```python
from build123d import *

# Parameters (mm, degrees)
PAD_DEPTH       = 3
SKETCH001_R     = 8.6
POCKET_DEPTH    = 3.001
SKETCH002_W     = 50
SKETCH002_H     = 6
PAD001_DEPTH    = 6
SKETCH003_W     = 5
SKETCH003_H     = 4.5
POCKET001_DEPTH = 6


with BuildPart() as part:
    # Sketch → Pad (new body)
    with BuildSketch(Plane.XZ):
        with BuildLine():
            Line((-24, -25), (-24, -24))
            Line((-24, -24), (-23, -24))
            Line((-23, -24), (-23, -17))
            Line((-23, -17), (-26.5, -17))
            Line((-26.5, -17), (-26.5, -14))
            Line((-26.5, -14), (-23.5, -14))
            Line((-23.5, -14), (-23.5, 0))
            Line((-23.5, 0), (-25, 0))
            Line((-25, 0), (-25, 30))
            Line((-25, 30), (25, 30))
            Line((25, 30), (25, 0))
            Line((25, 0), (23.5, 0))
            Line((23.5, 0), (23.5, -14))
            Line((23.5, -14), (26.5, -14))
            Line((26.5, -14), (26.5, -17))
            Line((26.5, -17), (23, -17))
            Line((23, -17), (23, -24))
            Line((23, -24), (24, -24))
            Line((24, -24), (24, -25))
            ThreePointArc((19, -21), (20.983324, -23.645845), (24, -25))
            Line((19, -3), (19, -21))
            Line((14, -3), (19, -3))
            Line((14, -18), (14, -3))
            Line((-14, -18), (14, -18))
            Line((-14, -3), (-14, -18))
            Line((-19, -3), (-14, -3))
            Line((-19, -21), (-19, -3))
            ThreePointArc((-24, -25), (-21.025722, -23.592847), (-19, -21))
        make_face()
    extrude(amount=PAD_DEPTH)

    # Sketch001 (on Face30 of Pad) → Pocket (cut, through all)
    with BuildSketch(Plane.XZ.offset(3)):
        with Locations((-13, 12)):
            Circle(SKETCH001_R)
        with Locations((13, 12)):
            Circle(SKETCH001_R)
    extrude(amount=-POCKET_DEPTH, mode=Mode.SUBTRACT)

    # Sketch002 (on Face5 of Pocket) → Pad001 (join)
    with BuildSketch(Plane.XZ.offset(3)):
        with Locations((0, 27)):
            Rectangle(SKETCH002_W, SKETCH002_H)
    extrude(amount=PAD001_DEPTH)

    # Sketch003 (on Face35 of Pad001) → Pocket001 (cut)
    with BuildSketch(Plane(origin=(0, 0, 30), x_dir=(-1, 0, 0), z_dir=(0, 0, 1))):
        with Locations((-20, 5.25)):
            Rectangle(SKETCH003_W, SKETCH003_H)
        with Locations((20, 5.25)):
            Rectangle(SKETCH003_W, SKETCH003_H)
    extrude(amount=-POCKET001_DEPTH, mode=Mode.SUBTRACT)


solid = part.part
```
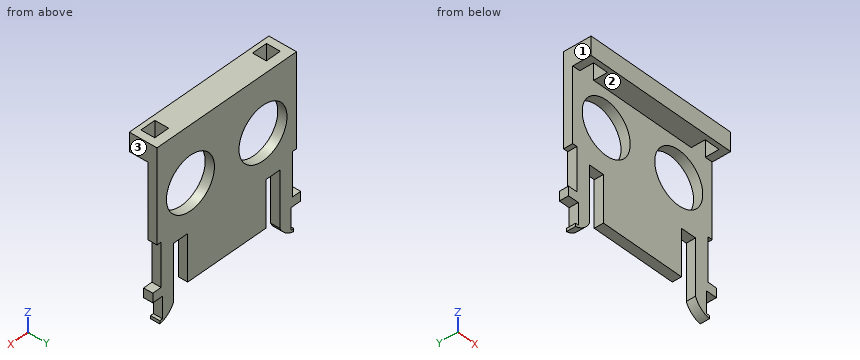
Work out the finished part from the listing and answer in its coordinate system (mm). Face numbers are marked on the shaded views. A direction names the side the tool comes from. Give positions to 0.01 mm unless a question says otherwise; leave off trailing zeros. Order: outer loops, then holes, each group sorted by start corner. A loop starts at its lowest first (then second) coordinate and runs counter-clockwise, first axis right, second up. Notation, with made-up numbers: (31, -35.5) -> (45, -35.5) arc R24 cw to (45, -20.5) -> close; hole circle Ø3 at (31.25, -13). An arc over 180 degrees is marked (long way). Answer as CSV lines item,"result". Start each with the question number.
(1) Consider line 1 along X through (y, z) = (-3.25, 27); line 2 along Z through (x, y) = (-13, -1); line 3 along Y through (x, z) = (5.5, -6.5). Determine where each line is inside the solid, lowest interval first.
(2) Each of these flat-tipped pins is pushed along its axis until it touches: pin 1 Ø2.5 at (x, y) = (15.5, -2) entering from -Z; pin 2 Ø1.5 at (x, z) = (-7, 18.5) entering from -Y; pin 3 Ø3.5 at (y, z) = (-5.5, 25.5) entering from +X. Where does it stop, or does it pass through?
(3) Which of the six approach directions +Z, -Z, +X, -X, +Y, -Y give full straight-line access (tool end or side, diameter ignored) to the marked faces 1, 2 and 3?
(4) Section A-A, the plane y = -4.5 is taken. Write down the section's boundary in (x, z), plus the area to 3 significant figures.
(5) Section D-D, the plane x = 8 is taken. Write down the section's boundary in (y, z), plus the area to 3 significant figures.
(6) Section C-C, the plane z = -11.5 is taken. Write down the section's boundary in (x, y).
(7) Section B-B, the plane x = -13 is taken. Write down the section's boundary in (y, z).
Entries:
1,line 1,"-25 to -22.5, -17.5 to 17.5, 22.5 to 25"
1,line 2,"-18 to 3.4, 20.6 to 30"
1,line 3,"-3 to 0"
2,pin 1,"z = -3"
2,pin 2,"y = -3"
2,pin 3,"x = 25"
3,face 1,"+Z, -X, +Y, -Y"
3,face 2,"-Z, +X, -X, -Y"
3,face 3,"+Z, +X, +Y, -Y"
4,outline,"(-25, 24) -> (-22.5, 24) -> (-22.5, 30) -> (-25, 30) -> close; (-17.5, 24) -> (17.5, 24) -> (17.5, 30) -> (-17.5, 30) -> close; (22.5, 24) -> (25, 24) -> (25, 30) -> (22.5, 30) -> close"
4,area,"240 mm²"
5,outline,"(-9, 24) -> (-3, 24) -> (-3, 19) -> (0, 19) -> (0, 30) -> (-9, 30) -> close; (-3, -18) -> (0, -18) -> (0, 5) -> (-3, 5) -> close"
5,area,"138 mm²"
6,outline,"(-23.5, -3) -> (-19, -3) -> (-19, 0) -> (-23.5, 0) -> close; (-14, -3) -> (14, -3) -> (14, 0) -> (-14, 0) -> close; (19, -3) -> (23.5, -3) -> (23.5, 0) -> (19, 0) -> close"
7,outline,"(-9, 24) -> (-3, 24) -> (-3, 20.6) -> (0, 20.6) -> (0, 30) -> (-9, 30) -> close; (-3, -18) -> (0, -18) -> (0, 3.4) -> (-3, 3.4) -> close"
